Source: CAD feature listing. Evaluate the final solid. Frame: model axes, mm. Round coordinates to 2 decimals unless told otherwise and drop trailing zeros. Loops run counter-clockwise (first coordinate to the right, second up) from the corner with the lowest first, then second, coordinate; pieces in that order, holes last. Notation, with made-up numbers: (-12, -4.75) - (26, -4.75) arc R29 cw to (26, 34.25) - close; hole circle Ø6 at (-23, 58). An arc over 180 degrees is marked (long way). One line per question, with ' | ' between items. Start each with the question number.
1. Ray query, line 1 (Z direction, x = 0, y = -0.7); line 2 (Z direction, x = 1, y = -0.2); line 3 (X direction, y = -1.35, z = -8.5). Return the intervals inside material, ascending.
2. Cut plane D-D (z = -18). Return loops of the section in (x, y).
3. Cut plane B-B (x = 24). Return loops of the section in (y, z), then the cut area to 3 significant figures.
4. Mould query, pull axis Z, two halves, no side actions, for faces 1 (the flat face through (-15, 0, -26)), 2 (the cylindrical face through (-5.077, -0.986, 38.668)), 3 (the cylindrical face through (30.5, -1.01, -19.05)). Classes: pulls with the +Z half, pulls with the -Z half, needs draft (parallel to the pull), parting line crosses it, or undercut.
5. Cut plane A-A (z = 36). Return loops of the section in (x, y).
6. Cut plane C-C (y = -1.55). Return loops of the section in (x, z) (3 decimals).
7. Pin query (flat end, axial travel): pin 1 (2 mm diameter, centred on x = -31.18, z = -18, fed in from +Y). Return the tip coordinate at first contact, or that it passes through.
```python
from build123d import *

# Parameters (mm, degrees)
F0_R            = 39
F0_R_2          = 29
F1_DEPTH        = 2
F2_R            = 1.25
F3_DEPTH        = 2.001
F3_COPIES_COUNT = 6


# Not quite as in the source:
# - a pattern or mirror of a feature is missing from the dataset's text; its kind, count and spacing are read off the source's solid


with BuildPart() as f1:
    # F0 (on Front) → F1 (new body)
    with BuildSketch(Plane.XZ):
        Circle(F0_R)
        Circle(F0_R_2, mode=Mode.SUBTRACT)
    extrude(amount=F1_DEPTH)

    # F2 (on face) → F3 (cut, through all)
    with BuildSketch(Plane.XZ.offset(2)):
        with Locations((31.1769145362, 18)):
            Circle(F2_R)
    f3 = extrude(amount=-F3_DEPTH, mode=Mode.SUBTRACT)

    # F3_copies: F3 ×6 about axis
    f3_copies_axis = Axis((0, 0, 0), (0, 1, 0))
    for i in range(1, F3_COPIES_COUNT):
        add(f3.rotate(f3_copies_axis, i * 360 / F3_COPIES_COUNT), mode=Mode.SUBTRACT)


solid = f1.part
```
Answers follow:
1) line 1: z = -39 to -37.25, -34.75 to -29, 29 to 34.75, 37.25 to 39 | line 2: z = -38.99 to -36.75, -35.25 to -28.98, 28.98 to 35.25, 36.75 to 38.99 | line 3: x = -38.06 to -27.73, 27.73 to 38.06
2) outline: (-34.6, -2) - (-32.43, -2) - (-32.43, 0) - (-34.6, 0) - close; (-29.93, -2) - (-22.74, -2) - (-22.74, 0) - (-29.93, 0) - close; (22.74, -2) - (29.93, -2) - (29.93, 0) - (22.74, 0) - close; (32.43, -2) - (34.6, -2) - (34.6, 0) - (32.43, 0) - close
3) outline: (-2, -30.74) - (0, -30.74) - (0, -16.28) - (-2, -16.28) - close; (-2, 16.28) - (0, 16.28) - (0, 30.74) - (-2, 30.74) - close | area: 57.8 mm2
4) face 1: needs draft | face 2: parting line crosses it | face 3: undercut
5) outline: (-15, -2) - (-1.25, -2) - (-1.25, 0) - (-15, 0) - close; (1.25, -2) - (15, -2) - (15, 0) - (1.25, 0) - close
6) outline: circle Ø78 at (0, 0); hole circle Ø2.5 at (-31.177, -18); hole circle Ø2.5 at (-31.177, 18); hole circle Ø58 at (0, 0); hole circle Ø2.5 at (0, -36); hole circle Ø2.5 at (0, 36); hole circle Ø2.5 at (31.177, -18); hole circle Ø2.5 at (31.177, 18)
7) pin 1: passes through
